```python
from build123d import *

# Parameters (mm, degrees)
SALIENTE_EXTRUIR1_DEPTH = 50
CROQUIS2_R              = 1.5
CORTAR_EXTRUIR1_DEPTH   = 10
CORTAR_EXTRUIR2_START   = -10
CROQUIS3_R              = 1.5
CORTAR_EXTRUIR2_DEPTH   = 10


with BuildPart() as part:
    # Croquis1 → Saliente-Extruir1 (new body)
    with BuildSketch(Plane(origin=(0, 0, 0), x_dir=(1, 0, 0), z_dir=(0, 1, 0))):
        Polygon((3.1, 0), (1.55, 2.684678752), (-1.55, 2.684678752), (-3.1, 0), (-1.55, -2.684678752), (1.55, -2.684678752), align=None)
    extrude(amount=SALIENTE_EXTRUIR1_DEPTH)

    # Croquis2 → Cortar-Extruir1 (cut)
    with BuildSketch(Plane(origin=(0, 50, 0), x_dir=(1, 0, 0), z_dir=(0, 1, 0))):
        with Locations(Location((0, 0, 0), (0, 0, 270))):
            Circle(CROQUIS2_R)
    extrude(amount=-CORTAR_EXTRUIR1_DEPTH, mode=Mode.SUBTRACT)

    # Croquis3 → Cortar-Extruir2 (cut)
    with BuildSketch(Plane.XZ.offset(CORTAR_EXTRUIR2_START)):
        with Locations(Location((0, 0, 0), (0, 0, 90))):
            Circle(CROQUIS3_R)
    extrude(amount=CORTAR_EXTRUIR2_DEPTH, mode=Mode.SUBTRACT)


solid = part.part
```
Geometry: final body of the model. Coordinates: model frame, mm. A direction names the side the tool comes from. Round coordinates to 2 decimals unless told otherwise and drop trailing zeros. Loops run counter-clockwise (first coordinate to the right, second up) from the corner with the lowest first, then second, coordinate; pieces in that order, holes last. Notation, with made-up numbers: (24.25, 27) -> (43.25, 27) arc R16 ccw to (43.25, 38) -> close; hole circle Ø8 at (-22, 30). An arc over 180 degrees is marked (long way). Use one line per item in the form item = value.
Item 1: Contact query for flat-ended pins moving along their axis: pin 1 Ø2 at (x, z) = (-1, 1.5) entering from -Y; pin 2 Ø3 at (y, z) = (35.5, 1) entering from +X; pin 3 Ø2.5 at (x, z) = (0, 0) entering from +Y. Output: stop coordinate, or through.
Evaluation:
pin_1 = 0
pin_2 = 3.1
pin_3 = 40
Item 2: Cut plane D-D on y = 24.5. Output: boundary loops of the cut face in (x, z), then the cut area to 3 significant figures.
Evaluation:
outline = (-3.1, 0) -> (-1.55, -2.68) -> (1.55, -2.68) -> (3.1, 0) -> (1.55, 2.68) -> (-1.55, 2.68) -> close
area = 25.0 mm2
Item 3: Cut plane B-B on x = 0. Output: boundary loops of the cut face in (y, z).
Evaluation:
outline = (0, -2.68) -> (50, -2.68) -> (50, -1.5) -> (40, -1.5) -> (40, 1.5) -> (50, 1.5) -> (50, 2.68) -> (0, 2.68) -> (0, 1.5) -> (10, 1.5) -> (10, -1.5) -> (0, -1.5) -> close
Item 4: Cut plane C-C on z = 0.8. Output: boundary loops of the cut face in (x, y).
Evaluation:
outline = (-2.64, 0) -> (-1.27, 0) -> (-1.27, 10) -> (1.27, 10) -> (1.27, 0) -> (2.64, 0) -> (2.64, 50) -> (1.27, 50) -> (1.27, 40) -> (-1.27, 40) -> (-1.27, 50) -> (-2.64, 50) -> close
Item 5: Access query for faces 4 (the flat face through (0, 10, 0)), 5 (the flat face through (0, 40, 0)), 6 (the flat face through (1.3, 0, -1.2)). Directions: +Z, -Z, +X, -X, +Y, -Y. A direction counts if a zero-diameter tool reaches every point of the face in a straight line with its end or side. Return the directions, or none.
Evaluation:
face_4 = -Y
face_5 = +Y
face_6 = +Z, -Z, +X, -X, -Y
Item 6: Material intervals for probe 1 along X at (y, z) = (47.25, 0); probe 2 along X at (y, z) = (3, -1); probe 3 along Y at (x, z) = (-0.5, -0.8), sorted ascending.
Evaluation:
probe_1 = -3.1 to -1.5, 1.5 to 3.1
probe_2 = -2.52 to -1.12, 1.12 to 2.52
probe_3 = 10 to 40
Item 7: Draft query along X for faces 1 (the cylindrical face through (0.45, 45.07, 1.43)), 2 (the flat face through (-2.314, 24.65, -1.361)), 3 (the flat face through (0, 25, 2.685)). Return one class per face: released by +X, released by -X, zero draft, split by the parting line, or undercut.
Evaluation:
face_1 = undercut
face_2 = released by -X
face_3 = zero draft
Item 8: Cut plane A-A on y = 44.5. Output: boundary loops of the cut face in (x, z).
Evaluation:
outline = (-3.1, 0) -> (-1.55, -2.68) -> (1.55, -2.68) -> (3.1, 0) -> (1.55, 2.68) -> (-1.55, 2.68) -> close; hole circle Ø3 at (0, 0)
